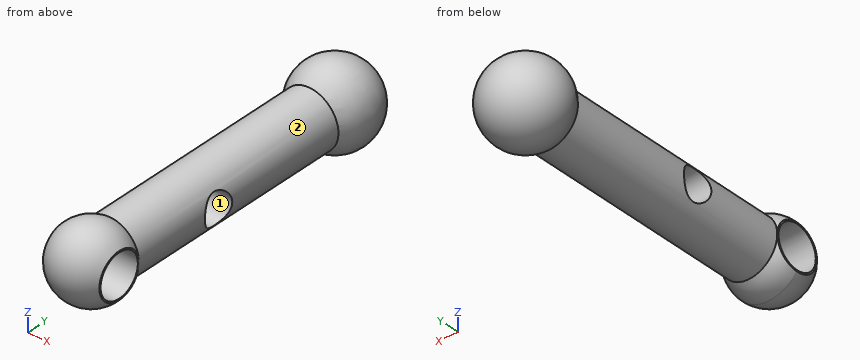
from build123d import *
from build123d.topology import SkipClean

# Parameters (mm, degrees)
SKETCH3_R           = 4.7625
CUT_EXTRUDE1_DEPTH  = 22.86
BOSS_EXTRUDE1_START = 5.08
SKETCH4_R           = 6.35
BOSS_EXTRUDE1_DEPTH = 57.15
SKETCH6_R           = 3.4925
CUT_EXTRUDE2_DEPTH  = 75.063978424


with BuildPart() as part:
    # Sketch1 → Revolve1 (revolve)
    with BuildSketch(Plane(origin=(0, 0, 0), x_dir=(1, 0, 0), z_dir=(0, 1, 0))):
        with BuildLine():
            Line((0, 0), (0, -5.08))
            Line((0, -5.08), (12.7, -5.08))
            Line((12.7, -5.08), (12.7, 0))
            ThreePointArc((12.7, 0), (6.35, 3.051967782), (0, 0))
        make_face()
    revolve(axis=Axis((0, 0, 5.08), (1, 0, 0)))

    # Sketch3 → Cut-Extrude1 (cut)
    with BuildSketch(Plane.ZY):
        with Locations((5.08, 0)):
            Circle(SKETCH3_R)
    extrude(amount=-CUT_EXTRUDE1_DEPTH, mode=Mode.SUBTRACT)

    # Sketch4 → Boss-Extrude1 (add)
    with SkipClean():  # the faces are left unmerged after this step: merging them gives an invalid solid
        with BuildSketch(Plane(origin=(0, 0, 0), x_dir=(1, 0, 0), z_dir=(0, 1, 0)).offset(BOSS_EXTRUDE1_START)):
            with Locations(Location((6.35, -5.08, 0), (0, 0, 180))):
                Circle(SKETCH4_R)
        extrude(amount=BOSS_EXTRUDE1_DEPTH)

    # Sketch5 → Revolve2 (revolve)
    with SkipClean():  # the faces are left unmerged after this step: merging them gives an invalid solid
        with BuildSketch(Plane(origin=(0, 62.23, 0), x_dir=(1, 0, 0), z_dir=(0, 1, 0))):
            with BuildLine():
                Line((6.35, 3.81), (6.35, -13.97))
                ThreePointArc((6.35, -13.97), (15.24, -5.08), (6.35, 3.81))
            make_face()
        revolve(axis=Axis((6.35, 62.23, -3.81), (0, 0, 1)))

    # Sketch6 → Cut-Extrude2 (cut, through all)
    with SkipClean():  # the faces are left unmerged after this step: merging them gives an invalid solid
        with BuildSketch(Plane(origin=(0, 0, 0), x_dir=(0, 0, -1), z_dir=(1, 0, 0))):
            with Locations(Location((-5.08, 25.4, 0), (0, 0, 180))):
                Circle(SKETCH6_R)
        extrude(amount=CUT_EXTRUDE2_DEPTH, mode=Mode.SUBTRACT)


solid = part.part
Verification items for the finished model (mm, model axes). Face numbers are marked on the shaded views. Coordinates: 2 decimals unless noted, no trailing zeros. Loops run counter-clockwise (first coordinate to the right, second up) from the corner with the lowest first, then second, coordinate; pieces in that order, holes last. Notation, with made-up numbers: M 8.25,74.5 L 26.25,74.5 A21 ccw 26.25,82.5 Z; hole C 89.5,-21 d11. An arc over 180 degrees is marked long. One line per item, written item: value.
1. Section check B-B on x = 6.35. Record the cut outline in (y, z) (1 decimal).
Answers follow:
outline: M 5.1,-1.3 L 56,-1.3 A8.9 ccw long 56,11.4 L 5.1,11.4 A8.1 ccw long Z; hole C 0,5.1 d9.5; hole C 25.4,5.1 d7
2. Section check C-C on y = 36.5. Record the cut outline in (x, z), plus the area to 3 significant figures.
Answers follow:
outline: C 6.35,5.08 d12.7
area: 127 mm^2
3. Material ranges on line 1 along Z through (x, y) = (6, 25.4); line 2 along Y through (x, z) = (12.5, 7); line 3 along Y through (x, z) = (10, 5.08), recorded low to high. Write a range as from..to.
Answers follow:
line 1: -1.26..1.59, 8.57..11.42
line 2: -4.96..-4.36, 4.36..4.96, 56.1..68.36
line 3: -7.27..-4.76, 4.76..21.91, 28.89..70.34
4. Section check A-A on z = 6. Record the cut outline in (x, y).
Answers follow:
outline: M 0,-5 A8.08 ccw 12.7,-5 L 12.7,-4.67 L 0,-4.67 Z; M 0,4.67 L 12.7,4.67 L 12.7,5 A8.08 ccw 12.63,5.08 L 12.63,22.03 L 0.07,22.03 L 0.07,5.08 A8.08 ccw 0,5 Z; M 0.07,28.77 L 12.63,28.77 L 12.63,56.01 A8.84 ccw long 0.07,56.01 Z
5. Gauge pin test, flat ends, axial feed: P1, Ø5, axis at x = 11, y = 51, coming from the +Z side; P2, Ø10, axis at y = 25, z = -0.5, coming from the -X side; P3, Ø3, axis at y = -0.5, z = 3.5, coming from the -X side; P4, Ø1.5, axis at y = 8, z = 5.5, coming from the +X side. Record the tip position at first contact, or that the pin passes through.
Answers follow:
P1: z = 11.05
P2: x = 0.16
P3: through
P4: x = 12.7
6. Section check D-D on y = 25.4. Record the cut outline in (x, z).
Answers follow:
outline: M 1.05,1.59 A6.35 ccw 11.65,1.59 Z; M 1.05,8.57 L 11.65,8.57 A6.35 ccw Z
7. Mould release check, pull along Z, two halves, no side actions. Record for the marked faces 1 and 2: pulls with the +Z half, pulls with the -Z half, needs draft (parallel to the pull), parting line crosses it, or undercut.
Answers follow:
face 1: undercut
face 2: parting line crosses it
